from build123d import *

# Parameters (mm, degrees)
SKETCH1_R               = 1.75
SKETCH1_W               = 53
SKETCH1_H               = 30
BOSS_EXTRUDE1_DEPTH     = 2
BOSS_EXTRUDE2_OUTLINE_R = 1.75
BOSS_EXTRUDE2_DEPTH     = 11.5
SKETCH3_R               = 1.75
SKETCH3_W               = 53
SKETCH3_H               = 30
BOSS_EXTRUDE3_DEPTH     = 2
BOSS_EXTRUDE4_DEPTH     = 6
BOSS_EXTRUDE5_DEPTH     = 6
SKETCH7_W               = 3.3
SKETCH7_H               = 5
CUT_EXTRUDE3_DEPTH      = 2
SKETCH9_W               = 55
SKETCH9_H               = 5.5
CUT_EXTRUDE5_DEPTH      = 14
SKETCH10_W              = 5.5
SKETCH10_H              = 11.5
BOSS_EXTRUDE6_DEPTH     = 55
BOSS_EXTRUDE8_DEPTH     = 8.5
CUT_EXTRUDE6_DEPTH      = 3
SKETCH15_R              = 1.3
CUT_EXTRUDE7_DEPTH      = 8


# Read off the part's stored shape, not the designer's step: Boss-Extrude2
with BuildPart() as part:
    # Sketch1 → Boss-Extrude1 (new body)
    with BuildSketch(Plane(origin=(0, 0, 0), x_dir=(1, 0, 0), z_dir=(0, 1, 0))):
        Polygon((0, 0), (23.2, 0), (23.2, -4.55), (20.8, -4.55), (20.8, -10), (28.65, -10), (28.65, -4.55), (71.7, -4.55), (71.7, 0), (83, 0), (83, -22.35), (83, -30.15), (83, -55), (72.2, -55), (72.2, -50.45), (33.2, -50.45), (33.2, -55), (0, -55), (0, -50.35), (19, -50.35), (19, -41.35), (0, -41.35), (0, -21.95), (17, -21.95), (17, -9.75), (0, -9.75), align=None)
        with Locations(Location((13.5, -4.85, 0), (0, 0, 270))):
            Circle(SKETCH1_R, mode=Mode.SUBTRACT)
        with Locations((47.3, -30.45)):
            Rectangle(SKETCH1_W, SKETCH1_H, mode=Mode.SUBTRACT)
    extrude(amount=BOSS_EXTRUDE1_DEPTH)

    # Boss-Extrude2 outline → Boss-Extrude2 (add)
    with BuildSketch(Plane.XZ):
        Polygon((0, 9.75), (0, 0), (20.8, 0), (20.8, 55), (0, 55), (0, 50.35), (19, 50.35), (19, 41.35), (0, 41.35), (0, 21.95), (17, 21.95), (17, 9.75), align=None)
        with Locations((13.5, 4.85)):
            Circle(BOSS_EXTRUDE2_OUTLINE_R, mode=Mode.SUBTRACT)
    extrude(amount=BOSS_EXTRUDE2_DEPTH)

    # Sketch3 → Boss-Extrude3 (add)
    with BuildSketch(Plane(origin=(0, 2, 0), x_dir=(1, 0, 0), z_dir=(0, 1, 0))):
        Polygon((23.2, 0), (0, 0), (0, -55), (33.2, -55), (33.2, -50.45), (72.2, -50.45), (72.2, -55), (83, -55), (83, 0), (71.7, 0), (71.7, -4.55), (28.65, -4.55), (28.65, -10), (20.8, -10), (20.8, -4.55), (23.2, -4.55), align=None)
        with Locations(Location((13.5, -4.85, 0), (0, 0, 90))):
            Circle(SKETCH3_R, mode=Mode.SUBTRACT)
        with Locations((47.3, -30.45)):
            Rectangle(SKETCH3_W, SKETCH3_H, mode=Mode.SUBTRACT)
    extrude(amount=BOSS_EXTRUDE3_DEPTH)

    # Sketch4 → Boss-Extrude4 (add)
    with BuildSketch(Plane.XY.offset(55)):
        Polygon((0, 4), (33.2, 4), (33.2, 0), (33.2, -1), (72.2, -1), (72.2, 0), (72.2, 4), (83, 4), (83, -11.5), (83, -16.5), (0, -16.5), (0, -11.5), align=None)
    extrude(amount=BOSS_EXTRUDE4_DEPTH)

    # Sketch5 → Boss-Extrude5 (add)
    with BuildSketch(Plane(origin=(0, 0, 0), x_dir=(-1, 0, 0), z_dir=(0, 0, -1))):
        Polygon((-23.2, 4), (-23.2, 0), (-23.2, -1), (-71.7, -1), (-71.7, 0), (-71.7, 4), (-83, 4), (-83, -11.5), (-83, -16.5), (0, -16.5), (0, -11.5), (0, 4), align=None)
    extrude(amount=BOSS_EXTRUDE5_DEPTH)

    # Sketch7 → Cut-Extrude3 (cut)
    with BuildSketch(Plane(origin=(0, 0, 55), x_dir=(-1, 0, 0), z_dir=(0, 0, -1))):
        with Locations((-14.15, -14)):
            Rectangle(SKETCH7_W, SKETCH7_H)
        with Locations((-68.85, -14)):
            Rectangle(SKETCH7_W, SKETCH7_H)
    extrude(amount=-CUT_EXTRUDE3_DEPTH, mode=Mode.SUBTRACT)

    # Sketch9 → Cut-Extrude5 (cut)
    with BuildSketch(Plane(origin=(20.8, 0, 0), x_dir=(0, 0, -1), z_dir=(1, 0, 0))):
        with Locations((-27.5, -8.75)):
            Rectangle(SKETCH9_W, SKETCH9_H)
    extrude(amount=-CUT_EXTRUDE5_DEPTH, mode=Mode.SUBTRACT)

    # Sketch10 → Boss-Extrude6 (add)
    with BuildSketch(Plane(origin=(0, 0, 55), x_dir=(-1, 0, 0), z_dir=(0, 0, -1))):
        with Locations((-80.25, -5.75)):
            Rectangle(SKETCH10_W, SKETCH10_H)
    extrude(amount=BOSS_EXTRUDE6_DEPTH)

    # Sketch12 → Boss-Extrude8 (add)
    with BuildSketch(Plane.XZ):
        Polygon((73.8, 45.45), (77.5, 45.45), (77.5, 50.45), (72.2, 50.45), (36.8, 50.45), (36.8, 45.45), align=None)
        Polygon((28.65, 10), (28.65, 4.55), (71.7, 4.55), (77.5, 4.55), (77.5, 15.45), (73.8, 15.45), (28.65, 15.45), align=None)
    extrude(amount=BOSS_EXTRUDE8_DEPTH)

    # Sketch14 → Cut-Extrude6 (cut)
    with BuildSketch(Plane.XZ.offset(16.5)):
        Polygon((79.299038106, 55.75), (80.598076211, 58), (79.299038106, 60.25), (76.700961894, 60.25), (75.401923789, 58), (76.700961894, 55.75), align=None)
        Polygon((6.299038106, 55.75), (3.700961894, 55.75), (2.401923789, 58), (3.700961894, 60.25), (6.299038106, 60.25), (7.598076211, 58), align=None)
        Polygon((3.700961894, -0.75), (2.401923789, -3), (3.700961894, -5.25), (6.299038106, -5.25), (7.598076211, -3), (6.299038106, -0.75), align=None)
        Polygon((76.700961894, -0.75), (79.299038106, -0.75), (80.598076211, -3), (79.299038106, -5.25), (76.700961894, -5.25), (75.401923789, -3), align=None)
    extrude(amount=-CUT_EXTRUDE6_DEPTH, mode=Mode.SUBTRACT)

    # Sketch15 → Cut-Extrude7 (cut)
    with BuildSketch(Plane.XZ.offset(16.5)):
        with Locations(Location((78, 58, 0), (0, 0, 270))):
            Circle(SKETCH15_R)
        with Locations(Location((5, 58, 0), (0, 0, 90))):
            Circle(SKETCH15_R)
        with Locations(Location((78, -3, 0), (0, 0, 90))):
            Circle(SKETCH15_R)
        with Locations(Location((5, -3, 0), (0, 0, 270))):
            Circle(SKETCH15_R)
    extrude(amount=-CUT_EXTRUDE7_DEPTH, mode=Mode.SUBTRACT)


solid = part.part
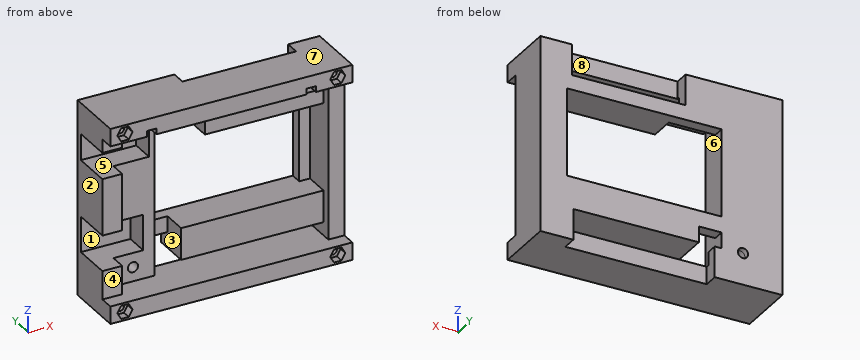
Can you work these out from the model? Positions are in its coordinate system, mm. Face numbers are marked on the shaded views. A direction names the side the tool comes from. Give positions to 0.01 mm unless a question says otherwise; leave off trailing zeros. Order: outer loops, then holes, each group sorted by start corner. A loop starts at its lowest first (then second) coordinate and runs counter-clockwise, first axis right, second up. Notation, with made-up numbers: M 75.25,-10 L 109.25,-10 A12 cw 109.25,8 Z; hole C 0,84 d1. An arc over 180 degrees is marked long. Use one line per item in the form item = value.
Item 1: If I drill on line 1 along Z through (x, y) = (55.5, -1.75); line 2 along Z through (x, y) = (78, -10.85); line 3 along Z through (x, y) = (10, -5.25), over which ranges is the centre line in solid material (lowest first)? Write a range as [from, to].
Values follow:
line_1 = [-6, 0], [4.55, 15.45], [45.45, 50.45], [55, 61]
line_2 = [-6, -4.3], [-1.7, 56.7], [59.3, 61]
line_3 = [-6, 9.75], [21.95, 41.35], [50.35, 61]
Item 2: If we section it at A-A, the plane y = -10.25: Write out the boundary of the cut face in (x, z).
Values follow:
outline = M 0,-6 L 83,-6 L 83,61 L 0,61 L 0,50.35 L 6.8,50.35 L 6.8,55 L 77.5,55 L 77.5,0 L 6.8,0 L 6.8,9.75 L 0,9.75 Z; M 0,21.95 L 6.8,21.95 L 6.8,41.35 L 0,41.35 Z; hole C 5,-3 d2.6; hole C 5,58 d2.6; hole C 78,-3 d2.6; hole C 78,58 d2.6
Item 3: If we section it at C-C, the plane z = 48: Write out the boundary of the cut face in (x, y).
Values follow:
outline = M 0,2 L 19,2 L 19,-6 L 20.8,-6 L 20.8,0 L 36.8,0 L 36.8,-8.5 L 77.5,-8.5 L 77.5,-11.5 L 83,-11.5 L 83,4 L 0,4 Z
Item 4: Thinking about a two-plate mould opening in X: for the marked faces 1, 2 and 3, which applies, pulls with the +X half, pulls with the -X half, needs draft (parallel to the pull), parting line crosses it, or undercut?
Values follow:
face_1 = needs draft
face_2 = pulls with the -X half
face_3 = undercut
Item 5: If we section it at B-B, the plane x = 13.5: Write out the boundary of the cut face in (y, z).
Values follow:
outline = M -16.5,-6 L 4,-6 L 4,3.1 L -6,3.1 L -6,0 L -16.5,0 Z; M -16.5,57 L -11.5,57 L -11.5,55 L -6,55 L -6,50.35 L 2,50.35 L 2,41.35 L -6,41.35 L -6,21.95 L 2,21.95 L 2,9.75 L -6,9.75 L -6,6.6 L 4,6.6 L 4,61 L -16.5,61 Z
Item 6: For the marked faces 4, 5, 6, 7 and 8, which set-ups out of +Z, -Z, +X, -X, +Y, -Y let a thin tool reach every point of the face, with its end or its side?
Values follow:
face_4 = +X, -X, -Y
face_5 = -X, -Y
face_6 = -Y
face_7 = +Z, +X, -X, +Y, -Y
face_8 = +Z, +Y
Item 7: Will these pins go through, and if not, where does the flat tip stop? pin 1 Ø6 at (x, z) = (79.5, 30) entering from -Y; pin 2 Ø3 at (x, z) = (78.5, 58.5) entering from -Y; pin 3 Ø12 at (x, z) = (57, 21) entering from -Y.
Values follow:
pin_1 = -11.5
pin_2 = -13.5
pin_3 = -8.5
